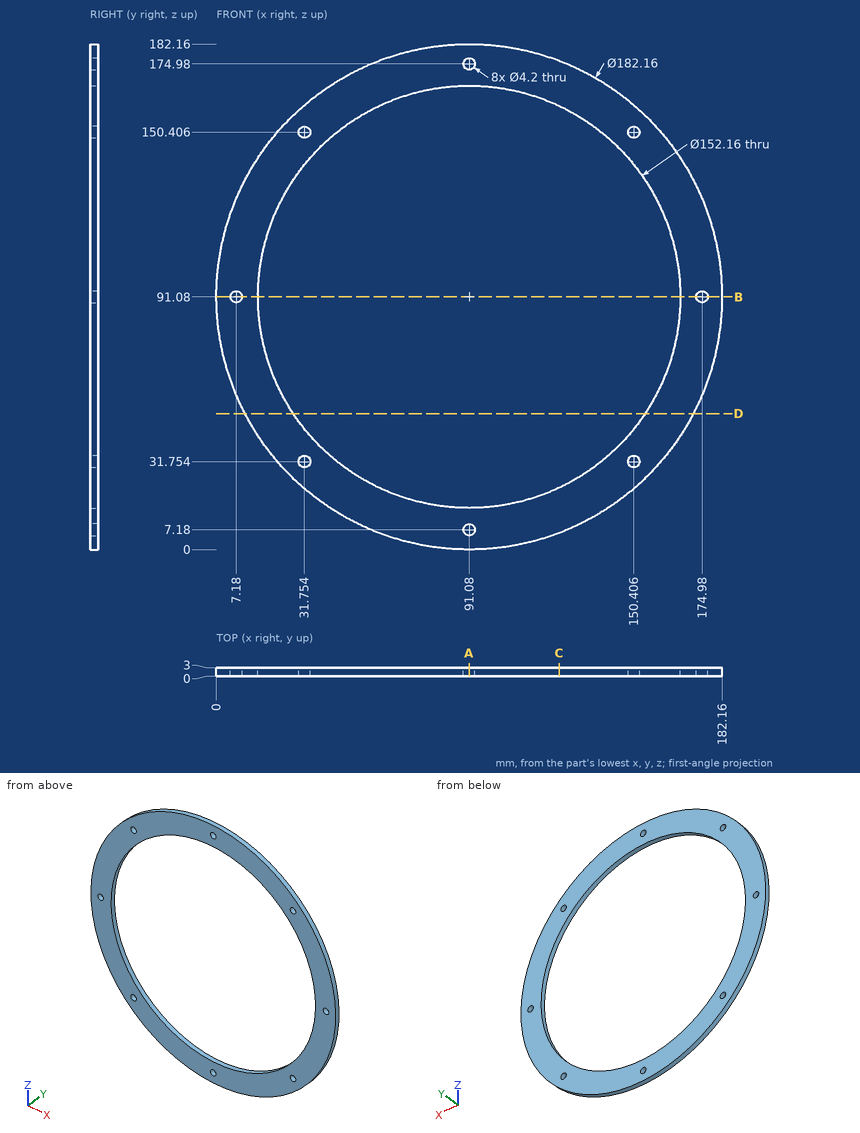
Geometry check sheet. Reference: drawing and pictorial views, mm from the part's lowest x, y, z. Give positions to 0.01 mm unless a question says otherwise; leave off trailing zeros. Loops run counter-clockwise (first coordinate to the right, second up) from the corner with the lowest first, then second, coordinate; pieces in that order, holes last. Notation, with made-up numbers: (2, 84.5) - (15, 84.5) arc R32 ccw to (15, 117.5) - close; hole circle Ø10 at (65.25, 43.25). An arc over 180 degrees is marked (long way). Use CSV: the item, a comma, the result in double quotes. Start each with the question number.
Q1. Section check A-A, the plane x = 91.08. Record the cut outline in (y, z), and give its area (3 significant figures).
Q2. Go/stop test with flat-tipped pins: pin 1 Ø3.5 at (x, z) = (31.75, 150.41) entering from -Y; pin 2 Ø1 at (y, z) = (0.5, 55.5) entering from -X; pin 3 Ø1.5 at (x, y) = (137.5, 2.5) entering from +Z; pin 4 Ø1.5 at (y, z) = (0.5, 108) entering from +X. Record where each tip stops, or that it passes through.
Q3. Section check B-B, the plane z = 91.08. Record the cut outline in (x, y).
Q4. Section check C-C, the plane x = 123.5. Record the cut outline in (y, z) (1 decimal).
Q5. Section check D-D, the plane z = 49. Record the cut outline in (x, y).
Q6. Scan lines: probe 1 along X at (y, z) = (0.8, 91.08); probe 2 along X at (y, z) = (2.75, 89.5) (1 decimal); probe 3 along Z at (x, y) = (149.5, 2.55) (1 decimal). Record each from-to range of solid material in increasing order. Write a range as from..to.
Findings below:
1,outline,"(0, 0) - (3, 0) - (3, 5.08) - (0, 5.08) - close; (0, 9.28) - (3, 9.28) - (3, 15) - (0, 15) - close; (0, 167.16) - (3, 167.16) - (3, 172.88) - (0, 172.88) - close; (0, 177.08) - (3, 177.08) - (3, 182.16) - (0, 182.16) - close"
1,area,"64.8 mm^2"
2,pin 1,"passes through"
2,pin 2,"stops at x = 7.03"
2,pin 3,"stops at z = 169.88"
2,pin 4,"stops at x = 180.71"
3,outline,"(0, 0) - (5.08, 0) - (5.08, 3) - (0, 3) - close; (9.28, 0) - (15, 0) - (15, 3) - (9.28, 3) - close; (167.16, 0) - (172.88, 0) - (172.88, 3) - (167.16, 3) - close; (177.08, 0) - (182.16, 0) - (182.16, 3) - (177.08, 3) - close"
4,outline,"(0, 6) - (3, 6) - (3, 22.3) - (0, 22.3) - close; (0, 159.9) - (3, 159.9) - (3, 176.2) - (0, 176.2) - close"
5,outline,"(10.3, 0) - (27.7, 0) - (27.7, 3) - (10.3, 3) - close; (154.46, 0) - (171.86, 0) - (171.86, 3) - (154.46, 3) - close"
6,probe 1,"x = 0..5.08, 9.28..15, 167.16..172.88, 177.08..182.16"
6,probe 2,"x = 0..5.8, 8.6..15, 167.1..173.6, 176.4..182.1"
6,probe 3,"z = 21.2..29.9, 33.6..42.3, 139.8..148.5, 152.3..161"
